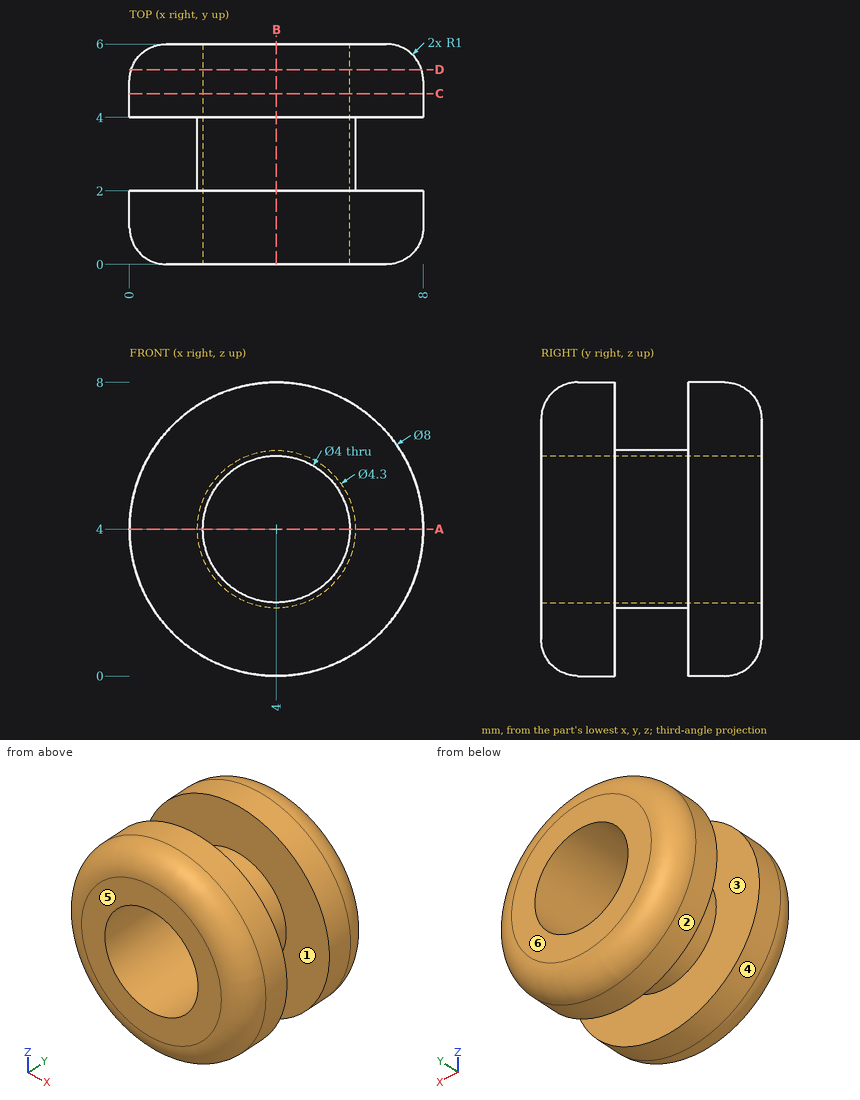
Geometry check sheet. Reference: drawing and pictorial views, mm from the part's lowest x, y, z. A direction names the side the tool comes from. Give positions to 0.01 mm unless a question says otherwise; leave off trailing zeros. Loops run counter-clockwise (first coordinate to the right, second up) from the corner with the lowest first, then second, coordinate; pieces in that order, holes last. Notation, with made-up numbers: M 17.5,87.5 L 29.5,87.5 A20 ccw 29.5,125.5 Z; hole C 30.25,6.25 d8. An arc over 180 degrees is marked long. One line per question, with ' | ' between items.
Item 1: Draft check along Y on the marked faces 3, 4, 5 and 6. Enter one of: +Y half, -Y half, draft (parallel to the pull), parting line (faces both ways), or undercut.
Completed:
face 3: undercut | face 4: draft | face 5: -Y half | face 6: +Y half
Item 2: Section check B-B, the plane x = 4. Record the cut outline in (y, z), plus the area to 3 significant figures.
Completed:
outline: M 0,1 A1 ccw 1,0 L 2,0 L 2,1.85 L 4,1.85 L 4,0 L 5,0 A1 ccw 6,1 L 6,2 L 0,2 Z; M 0,6 L 6,6 L 6,7 A1 ccw 5,8 L 4,8 L 4,6.15 L 2,6.15 L 2,8 L 1,8 A1 ccw 0,7 Z | area: 15.7 mm^2
Item 3: Tool access check on the marked faces 1 and 2. Record the directions out of +Z, -Z, +X, -X, +Y, -Y that give a thin tool (end or side, any length) a straight path to the whole face; none if there is none.
Completed:
face 1: none | face 2: +Y, -Y
Item 4: Section check D-D, the plane y = 5.3. Record the cut outline in (x, z), plus the area to 3 significant figures.
Completed:
outline: C 4,4 d7.91; hole C 4,4 d4 | area: 36.5 mm^2
Item 5: Section check C-C, the plane y = 4.65. Record the cut outline in (x, z), plus the area to 3 significant figures.
Completed:
outline: C 4,4 d8; hole C 4,4 d4 | area: 37.7 mm^2
Item 6: Thickness scan on line 1 (Y direction, x = 3, z = 6.25); line 2 (Z direction, x = 4, y = 4.05); line 3 (X direction, y = 4.4, z = 2.75). Record the ranges inside material, lowest first. Write a range as [from, to].
Completed:
line 1: y = [0, 2], [4, 6] | line 2: z = [0, 2], [6, 8] | line 3: x = [0.2, 2.44], [5.56, 7.8]
Item 7: Section check A-A, the plane z = 4. Record the cut outline in (x, y).
Completed:
outline: M 0,1 A1 ccw 1,0 L 2,0 L 2,6 L 1,6 A1 ccw 0,5 L 0,4 L 1.85,4 L 1.85,2 L 0,2 Z; M 6,0 L 7,0 A1 ccw 8,1 L 8,2 L 6.15,2 L 6.15,4 L 8,4 L 8,5 A1 ccw 7,6 L 6,6 Z
Item 8: Depth check by flat-ended pin: P1, Ø1.5, axis at x = 2.5, y = 5, coming from the -Z side; P2, Ø1.5, axis at y = 3, z = 6, coming from the -X side. Enter the tip coordinate at first touch or a pass-through.
Completed:
P1: stops at z = 0.07 | P2: stops at x = 2.25
